Verification items for this drawing (mm, ordinates from the low corner). A direction names the side the tool comes from. Coordinates: 2 decimals unless noted, no trailing zeros. Order: outer loops, then holes, each group sorted by start corner. A loop starts at its lowest first (then second) coordinate and runs counter-clockwise, first axis right, second up. Notation, with made-up numbers: M -23.5,80.5 L 24.5,80.5 A8 ccw 24.5,95.5 Z; hole C 54,-28 d11. An arc over 180 degrees is marked long. Answer as a JSON object with one key per item and string values. Group by question number.
(1) Gauge pin test, flat ends, axial feed: pin 1 Ø1.5 at (x, y) = (5.5, 15) entering from +Z; pin 2 Ø1 at (x, z) = (3.5, 1.5) entering from +Y. Record the tip position at first contact, or that the pin passes through.
(2) Material ranges on line 1 (Y direction, x = 7.25, z = 4.75); line 2 (Y direction, x = 1.75, z = 5.25); line 3 (X direction, y = 1.75, z = 5.5), recorded low to high.
(3) Cross-section at B-B (z = 4). Enter the section's corners in (x, y) (3 decimals), plus the area to 3 significant figures.
(4) Access from +Z, -Z, +X, -X, +Y, -Y to the whole of each face (thin tool, end or side, straight path). Record for the marked faces 1 and 2.
(5) Cross-section at A-A (x = 4). Enter the section's corners in (y, z) (3 decimals), plus the area to 3 significant figures.
(6) Cross-section at D-D (z = 7). Enter the section's corners in (x, y), plus the area to 3 significant figures.
(7) Cross-section at C-C (y = 17.25). Enter the section's corners in (x, z), plus the area to 3 significant figures.
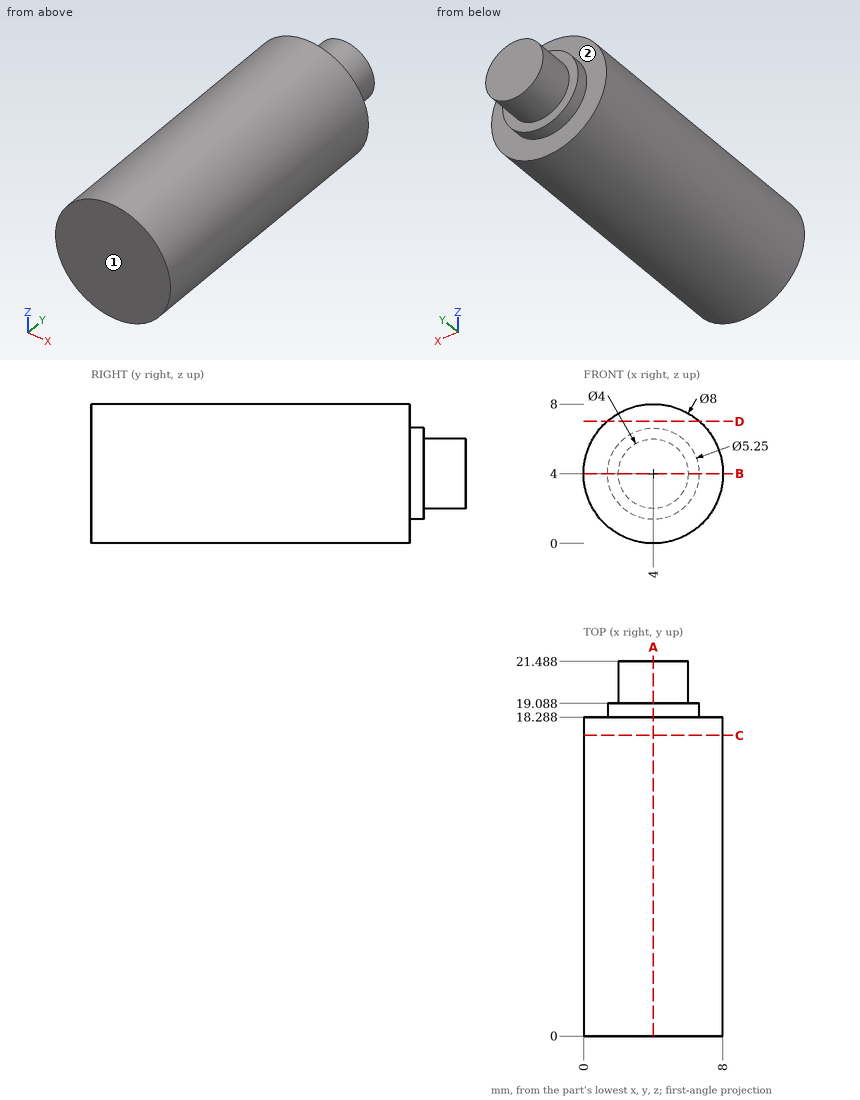
Taken from the geometry:
{
 "1": {"pin 1": "stops at z = 7.93", "pin 2": "stops at y = 19.09"},
 "2": {"line 1": "y = 0 to 18.29", "line 2": "y = 0 to 19.09", "line 3": "x = 0.29 to 7.71"},
 "3": {"outline": "M 0,0 L 8,0 L 8,18.288 L 6.625,18.288 L 6.625,19.088 L 6,19.088 L 6,21.488 L 2,21.488 L 2,19.088 L 1.375,19.088 L 1.375,18.288 L 0,18.288 Z", "area": "160 mm²"},
 "4": {"face 1": "+Z, -Z, +X, -X, -Y", "face 2": "+Y"},
 "5": {"outline": "M 0,0 L 18.288,0 L 18.288,1.375 L 19.088,1.375 L 19.088,2 L 21.488,2 L 21.488,6 L 19.088,6 L 19.088,6.625 L 18.288,6.625 L 18.288,8 L 0,8 Z", "area": "160 mm²"},
 "6": {"outline": "M 1.35,0 L 6.65,0 L 6.65,18.29 L 1.35,18.29 Z", "area": "96.8 mm²"},
 "7": {"outline": "C 4,4 d8", "area": "50.3 mm²"}
}
